For this review, take the finished solid that the model builds, in its own axes (mm). Face numbers are marked on the shaded views. A direction names the side the tool comes from. Give positions to 0.01 mm unless a question says otherwise; leave off trailing zeros. Loops run counter-clockwise (first coordinate to the right, second up) from the corner with the lowest first, then second, coordinate; pieces in that order, holes last.
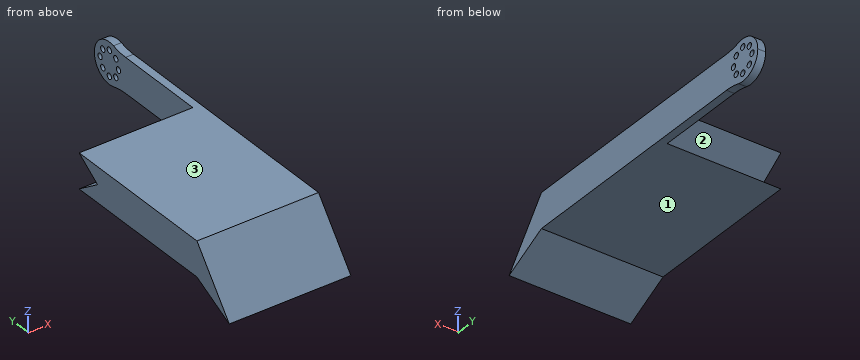
```python
from build123d import *

# Parameters (mm, degrees)
F2_DEPTH = 76.999998
F1_R     = 1.8542
F1_R_2   = 1.849996
F3_DEPTH = 4.99999
F4_R     = 38.1
F5_R     = 38.1


with BuildPart() as f2:
    # F0 (on Right) → F2 (new body)
    with BuildSketch(Plane.YZ):
        Polygon((60.006157, 31.522735), (-42.191276, 31.522735), (-70.230425, -4.425786), (-42.191276, 9.513999), (60.018324, 9.513999), (44.03463, 20.518491), align=None)
    extrude(amount=-F2_DEPTH)

    # F1 (on Right) → F3 (join)
    with BuildSketch(Plane.YZ):
        with BuildLine():
            ThreePointArc((145.413895, 20.522193), (138.69693, 31.902865), (125.487357, 31.522735))
            ThreePointArc((125.487357, 31.522735), (119.414457, 20.515007), (125.499524, 9.513999))
            ThreePointArc((125.499524, 9.513999), (138.703221, 9.144996), (145.413895, 20.522193))
        make_face()
        with Locations((132.414175, 12.526273)):
            Circle(F1_R, mode=Mode.SUBTRACT)
        with Locations((126.760205, 14.868224)):
            Circle(F1_R, mode=Mode.SUBTRACT)
        with Locations((138.068144, 14.868224)):
            Circle(F1_R, mode=Mode.SUBTRACT)
        with Locations((124.418255, 20.522193)):
            Circle(F1_R, mode=Mode.SUBTRACT)
        with Locations((140.410095, 20.522193)):
            Circle(F1_R, mode=Mode.SUBTRACT)
        with Locations((126.760205, 26.176162)):
            Circle(F1_R, mode=Mode.SUBTRACT)
        with Locations((138.070829, 26.178848)):
            Circle(F1_R_2, mode=Mode.SUBTRACT)
        with Locations((132.414175, 28.518113)):
            Circle(F1_R, mode=Mode.SUBTRACT)
        with BuildLine():
            Line((125.487357, 31.522735), (60.006157, 31.522735))
            Line((60.006157, 31.522735), (44.03463, 20.518491))
            Line((44.03463, 20.518491), (60.018324, 9.513999))
            Line((60.018324, 9.513999), (125.499524, 9.513999))
            ThreePointArc((125.499524, 9.513999), (119.414457, 20.515007), (125.487357, 31.522735))
        make_face()
    extrude(amount=-F3_DEPTH)

    # F4
    f4_edges = [f2.edges().sort_by_distance(p)[0] for p in [
        (-2.499995, 125.487357, 31.522735),
    ]]
    fillet(f4_edges, radius=F4_R)

    # F5
    f5_edges = [f2.edges().sort_by_distance(p)[0] for p in [
        (-2.499995, 125.499524, 9.513999),
    ]]
    fillet(f5_edges, radius=F5_R)


solid = f2.part
```
Item 1: Take a section at A-A on x = -64.5. Give the boundary of the cut face in (y, z).
Answer:
outline: (-70.23, -4.43) - (-42.19, 9.51) - (60.02, 9.51) - (44.03, 20.52) - (60.01, 31.52) - (-42.19, 31.52) - close
Item 2: Clearance check with flat-ended pins moving along their axes: pin 1 Ø8 at (y, z) = (118.5, 17.5) entering from -X; pin 2 Ø3 at (x, z) = (-32.5, 19) entering from +Y; pin 3 Ø8 at (x, y) = (-64, -1.5) entering from +Z. State where each tip first meets the part, or that it passes through.
Answer:
pin 1: stops at x = -5
pin 2: stops at y = 48.42
pin 3: stops at z = 31.52
Item 3: Take a section at C-C on y = 105. Give the boundary of the cut face in (x, z), and give its area (3 significant figures).
Answer:
outline: (-5, 9.51) - (0, 9.51) - (0, 31.52) - (-5, 31.52) - close
area: 110 mm2
Item 4: For L1, parallel to Z at x = -8, y = -21; L2, parallel to X at y = 116.5, z = 15; L3, parallel to Y at x = -69, z = 22.5, list the stretches that pass through material, from the lowest coordinate up.
Answer:
L1: z = 9.51 to 31.52
L2: x = -5 to 0
L3: y = -49.23 to 46.91
Item 5: Take a section at B-B on y = 27. Give the boundary of the cut face in (x, z), and give its area (3 significant figures).
Answer:
outline: (-77, 9.51) - (0, 9.51) - (0, 31.52) - (-77, 31.52) - close
area: 1,690 mm2
Item 6: Tool access review of the marked faces 1, 2 and 3: name each direction out of +Z, -Z, +X, -X, +Y, -Y from which nothing blocks a thin tool from reaching the whole face with its end or side.
Answer:
face 1: -Z, +X, -X
face 2: -X, +Y
face 3: +Z, +X, -X, -Y
